```python
from build123d import *
from OCP.BRepFilletAPI import BRepFilletAPI_MakeChamfer

# Parameters (mm, degrees)
SKIZZE1_R                       = 2
AUFSATZ_LINEAR_AUSTRAGEN1_DEPTH = 8
SKIZZE2_R                       = 2.375
AUFSATZ_LINEAR_AUSTRAGEN2_DEPTH = 11
FASE1_SIZE                      = 3
FASE1_SIZE2                     = 0.860236157
AUFSATZ_LINEAR_AUSTRAGEN3_DEPTH = 0.4
SKIZZE5_R                       = 0.509593562
SCHNITT_LINEAR_AUSTRAGEN1_DEPTH = 26.48056909


with BuildPart() as part:
    # Skizze1 → Aufsatz-Linear austragen1 (new body)
    with BuildSketch(Plane.XY):
        with BuildLine():
            Line((-13.199545584, 2.739250778), (-3.959262527, 8.28677743))
            ThreePointArc((-3.959262527, 8.28677743), (-2.720950124, 8.81839637), (-1.385638765, 9))
            Line((-1.385638765, 9), (0, 9))
            Line((0, 9), (2.77127753, 9))
            Line((2.77127753, 9), (6.43, 9))
            Line((6.43, 9), (6.43, 6.803437374))
            Line((6.43, 6.803437374), (13.199545584, 2.739250778))
            ThreePointArc((13.199545584, 2.739250778), (14.75, 0), (13.199545584, -2.739250778))
            Line((13.199545584, -2.739250778), (5.147247524, -7.573554859))
            ThreePointArc((5.147247524, -7.573554859), (0, -9), (-5.147247524, -7.573554859))
            Line((-5.147247524, -7.573554859), (-13.199545584, -2.739250778))
            ThreePointArc((-13.199545584, -2.739250778), (-14.75, 0), (-13.199545584, 2.739250778))
        make_face()
        with Locations((-11.555, 0)):
            Circle(SKIZZE1_R, mode=Mode.SUBTRACT)
        with Locations(Location((11.555, 0, 0), (0, 0, 180))):
            Circle(SKIZZE1_R, mode=Mode.SUBTRACT)
    extrude(amount=AUFSATZ_LINEAR_AUSTRAGEN1_DEPTH)

    # Skizze2 → Aufsatz-Linear austragen2 (add)
    with BuildSketch(Plane(origin=(0, 9, 0), x_dir=(1, 0, 0), z_dir=(0, 1, 0))):
        with Locations(Location((4.055, -2.375, 0), (0, 0, 90))):
            Circle(SKIZZE2_R)
    extrude(amount=AUFSATZ_LINEAR_AUSTRAGEN2_DEPTH)

    # Skizze3 → Schnitt-Rotation5 (revolve, cut)
    with BuildSketch(Plane(origin=(0, 0, 2.37), x_dir=(-1, 0, 0), z_dir=(0, 0, -1)), mode=Mode.PRIVATE) as schnitt_rotation5_sk:
        Polygon((-5.548619779, 20), (-5.548619779, 19.390425007), (-6.43, 14.45438156), (-5.871186885, 14.45438156), (-5.871186885, 9.618429672), (-6.43, 9), (-7.295904823, 9), (-6.993468517, 15.795841506), (-6.993468517, 20), align=None)
    revolve(schnitt_rotation5_sk.sketch.rotate(Axis((4.055, 22.337602527, 2.37), (0, -1, 0)), 0.060311358), axis=Axis((4.055, 22.337602527, 2.37), (0, -1, 0)), mode=Mode.SUBTRACT)

    # Fase1: one chamfer whose edges measure the first distance from different faces: ONE call of the kernel's chamfer builder (chamfer() names one face for all edges)
    fase1_edges_1 = [part.edges().sort_by_distance(p)[0] for p in [
        (14.75, 0, 8),
    ]]
    fase1_side_1 = [part.faces().sort_by_distance(p)[0] for p in [
        (14.75, 0, 4),
    ]]
    fase1_edges_2 = [part.edges().sort_by_distance(p)[0] for p in [
        (9.814772792, 4.771344076, 8),
    ]]
    fase1_side_2 = [part.faces().sort_by_distance(p)[0] for p in [
        (9.814772792, 4.771344076, 4),
    ]]
    fase1_edges_3 = [part.edges().sort_by_distance(p)[0] for p in [
        (6.43, 7.901718687, 8),
    ]]
    fase1_side_3 = [part.faces().sort_by_distance(p)[0] for p in [
        (6.43, 7.901718687, 4),
    ]]
    fase1_edges_4 = [part.edges().sort_by_distance(p)[0] for p in [
        (2.522180617, 9, 8),
    ]]
    fase1_side_4 = [part.faces().sort_by_distance(p)[0] for p in [
        (1.917072159, 9, 4.642485362),
    ]]
    fase1_edges_5 = [part.edges().sort_by_distance(p)[0] for p in [
        (-2.720950124, 8.81839637, 8),
    ]]
    fase1_side_5 = [part.faces().sort_by_distance(p)[0] for p in [
        (-2.720950124, 8.81839637, 4),
    ]]
    fase1_edges_6 = [part.edges().sort_by_distance(p)[0] for p in [
        (-8.579404056, 5.513014104, 8),
    ]]
    fase1_side_6 = [part.faces().sort_by_distance(p)[0] for p in [
        (-8.579404056, 5.513014104, 4),
    ]]
    fase1_edges_7 = [part.edges().sort_by_distance(p)[0] for p in [
        (-14.75, 0, 8),
    ]]
    fase1_side_7 = [part.faces().sort_by_distance(p)[0] for p in [
        (-14.75, 0, 4),
    ]]
    fase1_edges_8 = [part.edges().sort_by_distance(p)[0] for p in [
        (-9.173396554, -5.156402818, 8),
    ]]
    fase1_side_8 = [part.faces().sort_by_distance(p)[0] for p in [
        (-9.173396554, -5.156402818, 4),
    ]]
    fase1_edges_9 = [part.edges().sort_by_distance(p)[0] for p in [
        (0, -9, 8),
    ]]
    fase1_side_9 = [part.faces().sort_by_distance(p)[0] for p in [
        (0, -9, 4),
    ]]
    fase1_edges_10 = [part.edges().sort_by_distance(p)[0] for p in [
        (9.173396554, -5.156402818, 8),
    ]]
    fase1_side_10 = [part.faces().sort_by_distance(p)[0] for p in [
        (9.173396554, -5.156402818, 4),
    ]]
    fase1 = BRepFilletAPI_MakeChamfer(part.part.solid().wrapped)
    for e in fase1_edges_1:
        fase1.Add(FASE1_SIZE, FASE1_SIZE2, e.wrapped, fase1_side_1[0].wrapped)  # the first distance lies on this face
    for e in fase1_edges_2:
        fase1.Add(FASE1_SIZE, FASE1_SIZE2, e.wrapped, fase1_side_2[0].wrapped)  # the first distance lies on this face
    for e in fase1_edges_3:
        fase1.Add(FASE1_SIZE, FASE1_SIZE2, e.wrapped, fase1_side_3[0].wrapped)  # the first distance lies on this face
    for e in fase1_edges_4:
        fase1.Add(FASE1_SIZE, FASE1_SIZE2, e.wrapped, fase1_side_4[0].wrapped)  # the first distance lies on this face
    for e in fase1_edges_5:
        fase1.Add(FASE1_SIZE, FASE1_SIZE2, e.wrapped, fase1_side_5[0].wrapped)  # the first distance lies on this face
    for e in fase1_edges_6:
        fase1.Add(FASE1_SIZE, FASE1_SIZE2, e.wrapped, fase1_side_6[0].wrapped)  # the first distance lies on this face
    for e in fase1_edges_7:
        fase1.Add(FASE1_SIZE, FASE1_SIZE2, e.wrapped, fase1_side_7[0].wrapped)  # the first distance lies on this face
    for e in fase1_edges_8:
        fase1.Add(FASE1_SIZE, FASE1_SIZE2, e.wrapped, fase1_side_8[0].wrapped)  # the first distance lies on this face
    for e in fase1_edges_9:
        fase1.Add(FASE1_SIZE, FASE1_SIZE2, e.wrapped, fase1_side_9[0].wrapped)  # the first distance lies on this face
    for e in fase1_edges_10:
        fase1.Add(FASE1_SIZE, FASE1_SIZE2, e.wrapped, fase1_side_10[0].wrapped)  # the first distance lies on this face
    add(Compound.cast(fase1.Shape()), mode=Mode.REPLACE)

    # Skizze4 → Aufsatz-Linear austragen3 (add)
    with BuildSketch(Plane.XY.offset(5.63)):
        Polygon((-1.52, -12), (-2.02, -12), (-2.02, -5), (-0.52, -5), (-0.52, -12), (-1.02, -12), (-1.02, -18), (-1.52, -18), align=None)
        Polygon((-4.06, -12), (-4.56, -12), (-4.56, -5), (-3.06, -5), (-3.06, -12), (-3.56, -12), (-3.56, -18), (-4.06, -18), align=None)
        Polygon((3.56, -12), (3.56, -18), (4.06, -18), (4.06, -12), (4.56, -12), (4.56, -5), (3.06, -5), (3.06, -12), align=None)
        Polygon((1.02, -12), (1.02, -18), (1.52, -18), (1.52, -12), (2.02, -12), (2.02, -5), (0.52, -5), (0.52, -12), align=None)
    extrude(amount=-AUFSATZ_LINEAR_AUSTRAGEN3_DEPTH)

    # Skizze5 → Schnitt-Linear austragen1 (cut, through all)
    with BuildSketch(Plane.XY.offset(5.63)):
        with Locations((-4.56, -10.577193371)):
            Circle(SKIZZE5_R)
    extrude(amount=-SCHNITT_LINEAR_AUSTRAGEN1_DEPTH, mode=Mode.SUBTRACT)


solid = part.part
```
Here's how the part is built. I have some questions about the finished solid (model axes, mm). A direction names the side the tool comes from. Give positions to 0.01 mm unless a question says otherwise; leave off trailing zeros. Order: outer loops, then holes, each group sorted by start corner. A loop starts at its lowest first (then second) coordinate and runs counter-clockwise, first axis right, second up. Notation, with made-up numbers: (22.5, -21.75) - (26.5, -21.75) arc R22 cw to (26.5, 4.25) - close; hole circle Ø4 at (79.5, 67). An arc over 180 degrees is marked (long way). Answer as a JSON object with one key per item and string values. Group by question number.
Item 1: Please list where these lines run through material, in increasing order: probe 1 along Y at (x, z) = (13, 7.75); probe 2 along Y at (x, z) = (-10, 3); probe 3 along Y at (x, z) = (-3, 4.5).
Item 2: If we section it at D-D on x = -6: Please give me the cut outline in (y, z), and give its area (3 significant figures).
Item 3: For P1, Ø1.8, axis at y = 8, z = 3, coming from the +X side; P2, Ø2, axis at x = 7, z = 4.5, coming from the +Y side; P3, Ø1, axis at x = 3, y = 10.5, coming from the +Z side; P4, Ø6, axis at x = -11.5, y = -10.5, coming from the -Z side, each with a flat end and sliding along its axis, tell me the tip position at first contact or that it passes through.
Item 4: If we section it at B-B on x = 11.5: Please give me the cut outline in (y, z).
Item 5: If we mould it in two halves opening along X, with no side actions, what happens to faces 1 (the conical face through (2.696, 17.436, 3.614)), 2 (the cylindrical face through (14.75, 0.05, 2.46)), 3 (the cylindrical face through (9.647, -0.601, 3.944)), 4 (the flat face through (-1.3, -12.2, 5.63))? For each: pulls with the +X half, pulls with the -X half, needs draft (parallel to the pull), parting line crosses it, or undercut.
Item 6: If we section it at C-C on z = 6.5: Please give me the cut outline in (x, y) (3 decimals), and give its area (3 significant figures).
Item 7: Which directions (+Z, -Z, +X, -X, +Y, -Y) give clear straight access to the entire face, cutting with the end or side of a thin tool? Please do faces 5 (the flat face through (-3.8, -11.6, 5.63)), 6 (the flat face through (6.43, 8, 2)), 7 (the conical face through (14.314, 0.04, 6.521)).
Item 8: If we section it at A-A on y = 0: Please give me the cut outline in (x, z) (3 decimals), and give its area (3 significant figures).
Result set:
{
 "1": {"probe 1": "-1.92 to -1.38, 1.38 to 1.92", "probe 2": "-4.66 to -1.26, 1.26 to 4.66", "probe 3": "-8.54 to 8.73"},
 "2": {"outline": "(-7.06, 0) - (7.06, 0) - (7.06, 5) - (6.06, 8) - (-6.06, 8) - (-7.06, 5) - close", "area": "110 mm²"},
 "3": {"P1": "x = 6.43", "P2": "y = 9", "P3": "z = 4.1", "P4": "through"},
 "4": {"outline": "(-3.76, 0) - (-2, 0) - (-2, 8) - (-2.76, 8) - (-3.76, 5) - close; (2, 0) - (3.76, 0) - (3.76, 5) - (2.76, 8) - (2, 8) - close"},
 "5": {"face 1": "parting line crosses it", "face 2": "pulls with the +X half", "face 3": "undercut", "face 4": "needs draft"},
 "6": {"outline": "(-12.978, -2.37) - (-4.926, -7.205) arc R9.57 ccw to (4.926, -7.205) - (12.978, -2.37) arc R2.765 ccw to (12.978, 2.37) - (6, 6.56) - (6, 8.57) - (-1.386, 8.57) arc R4.57 ccw to (-3.738, 7.918) - (-12.978, 2.37) arc R2.765 ccw to start; hole circle Ø4 at (-11.555, 0); hole circle Ø4 at (11.555, 0)", "area": "303 mm²"},
 "7": {"face 5": "+Z, -X, -Y", "face 6": "+Z, -Z, +X, +Y", "face 7": "+Z, +X"},
 "8": {"outline": "(-14.75, 0) - (-13.555, 0) - (-13.555, 8) - (-13.89, 8) - (-14.75, 5) - close; (-9.555, 0) - (9.555, 0) - (9.555, 8) - (-9.555, 8) - close; (13.555, 0) - (14.75, 0) - (14.75, 5) - (13.89, 8) - (13.555, 8) - close", "area": "169 mm²"}
}
